Autodesk Fusion 360 part; units mm, degrees
sketch "Skizze1" plane through (0, 0, 0) normal (0, 0, 1) x (1, 0, 0)
  circle A0 centre (0, 0) radius 24.75
  circle A1 centre (0, 0) radius 21.75
  line L0 (-17.5, 13.5) -> (17.5, 13.5)
  line L1 (17.5, 13.5) -> (17.5, -13.5)
  line L2 (17.5, -13.5) -> (-17.5, -13.5)
  line L3 (-17.5, -13.5) -> (-17.5, 13.5)
  line L4 (-40, 0) -> (50, 0) construction
  line L5 (0, 45.7661) -> (0, -44.2339) construction
  line L6 (-16.0234, 16.5) -> (16.0234, 16.5)
  line L7 (20.5, 10.4283) -> (20.5, -10.4283)
  line L8 (16.0234, -16.5) -> (-16.0234, -16.5)
  line L9 (-20.5, -10.4283) -> (-20.5, 10.4283)
  arc A2 (6.5, 16.5) -> (-6.5, 16.5) centre (0, 16.5) ccw
  arc A3 (-6.6213, -16.5) -> (6.3787, -16.5) centre (-0.1213, -16.5) ccw
  arc A4 (-21.6357, 2.2272) -> (-21.6357, -2.2272) centre (-20.5, 0) ccw
  arc A5 (21.6357, -2.2272) -> (21.6357, 2.2272) centre (20.5, 0) ccw
  circle A6 centre (0, 0) radius 23
  line L10 (-14.5, -7.5) -> (14.5, -7.5)
  line L11 (14.5, -7.5) -> (14.5, 7.5)
  line L12 (14.5, 7.5) -> (-14.5, 7.5)
  line L13 (-14.5, 7.5) -> (-14.5, -7.5)
  line L14 (-15.5, 10.5) -> (15.5, 10.5)
  line L15 (15.5, 10.5) -> (15.5, -10.5)
  line L16 (15.5, -10.5) -> (-15.5, -10.5)
  line L17 (-15.5, -10.5) -> (-15.5, 10.5)
  dimension "d1" = 49.5
  dimension "d3" = 3
  dimension "d4" = 27
  dimension "d5" = 35
  dimension "d6" = 3
  dimension "d7" = 3
  dimension "d8" = 3
  dimension "d9" = 3
  dimension "d18" = 46
  dimension "d19" = 29
  dimension "d20" = 15
  dimension "d27" = 3
  dimension "d28" = 3
  dimension "d29" = 2
  dimension "d30" = 2
  dimension "d40" = 33
extrude "Extrusion5" add sketch "Skizze1" along normal blind 3 contours A1 L7 | A1 A5 | A1 L1 L7 | A1 L0 L1 L6 L7 A6 | A1 L1 L2 L7 L8 A6 | A1 L0 L6 | A1 L2 L8 | A1 L0 L3 L6 L9 A6 | A1 A2 | A1 A3 | A1 L2 L3 L8 L9 A6 | A1 L6 A2 | A1 L3 L9 | A1 L8 A3 | A1 L9 | A1 A4 picked at (0.4894, 18.2335) picked at (-0.6234, -18.2297)
extrude "Extrusion6" add sketch "Skizze1" along normal up to surface (1.5 mm away) from surface at 1.5 contours A1 L0 L1 L2 L3
hole "Bohrung1" at (0, 16.5, 0) at (20.5, 0, 0) at (-0.1213, -16.5, 0) at (-20.5, 0, 0) direction (0, 0, 1) diameter 2.5 end through all
fillet "Abrundung1" radius 7 4 edges at (-6.6213, -16.5, 1.5) (6.3787, -16.5, 1.5) (6.5, 16.5, 1.5) (-6.5, 16.5, 1.5)
Input: part model. Units: mm. Frame: model coordinates. A direction names the side the tool comes from. Give positions to 0.01 mm unless a question says otherwise; leave off trailing zeros. Order: outer loops, then holes, each group sorted by start corner. A loop starts at its lowest first (then second) coordinate and runs counter-clockwise, first axis right, second up.
Q1. Section B-B on x = 9. Output: boundary loops of the cut face in (y, z).
Checked values:
outline: (-16.93, 0) - (-13.5, 0) - (-13.5, 1.5) - (-10.5, 1.5) - (-10.5, 3) - (-16.93, 3) - close; (10.5, 1.5) - (13.5, 1.5) - (13.5, 0) - (16.98, 0) - (16.98, 3) - (10.5, 3) - close
Q2. Section C-C on y = -5.5. Output: boundary loops of the cut face in (x, z), and give its area (3 significant figures).
Checked values:
outline: (-21.04, 0) - (-17.5, 0) - (-17.5, 1.5) - (-15.5, 1.5) - (-15.5, 3) - (-21.04, 3) - close; (15.5, 1.5) - (17.5, 1.5) - (17.5, 0) - (21.04, 0) - (21.04, 3) - (15.5, 3) - close
area: 27.3 mm2
Q3. Section D-D on z = 0.7. State how many separate pieces and enclosed holes the cut face has, and give its area (3 significant figures).
Checked values:
separate pieces: 1
enclosed holes: 5
area: 520 mm2
Q4. Ray query, probe 1 along X at (y, z) = (0, 1.65); probe 2 along X at (y, z) = (7.5, 2.1); probe 3 along Y at (x, z) = (13, 1.4). Return the intervals inside material, ascending.
Checked values:
probe 1: x = -23 to -21.75, -19.25 to -15.5, 15.5 to 19.25, 21.75 to 23
probe 2: x = -20.5 to -15.5, 15.5 to 20.5
probe 3: y = -16.5 to -13.5, 13.5 to 16.5
Q5. Section A-A on y = 0. Output: boundary loops of the cut face in (x, z).
Checked values:
outline: (-23, 0) - (-21.75, 0) - (-21.75, 3) - (-23, 3) - close; (-19.25, 0) - (-17.5, 0) - (-17.5, 1.5) - (-15.5, 1.5) - (-15.5, 3) - (-19.25, 3) - close; (15.5, 1.5) - (17.5, 1.5) - (17.5, 0) - (19.25, 0) - (19.25, 3) - (15.5, 3) - close; (21.75, 0) - (23, 0) - (23, 3) - (21.75, 3) - close
Q6. Set-up query: faces 1 (the flat face through (-20.5, 9, 1)), 2 (the flat face through (-14, -16.5, 1)), 3 (the flat face through (20.5, 9, 1)). Return all of +Z, -Z, +X, -X, +Y, -Y with unobstructed straight access to the full face (end or side cutting, diameter ignored); none if empty.
Checked values:
face 1: +Z, -Z, -X, +Y
face 2: +Z, -Z, -X, -Y
face 3: +Z, -Z, +X, +Y
Q7. Draft query along Y for faces 4 (the cylindrical face through (-21.21, -4.82, 1.48)), 5 (the flat face through (-14, 16.5, 1)), 6 (the cylindrical face through (-0.18, -17.75, 1.52)). Return one class per face: +Y half, -Y half, draft (parallel to the pull), parting line (faces both ways), or undercut.
Checked values:
face 4: -Y half
face 5: +Y half
face 6: undercut
Q8. Contact query for flat-ended pins moving along their axis: pin 1 Ø1.5 at (y, z) = (8.5, 2) entering from -X; pin 2 Ø0.8 at (x, z) = (2, 2) entering from -Y; pin 3 Ø1.6 at (y, z) = (4.5, 2.5) entering from +X; pin 4 Ø2 at (x, y) = (-20.5, 0) entering from -Z. Output: stop coordinate, or through.
Checked values:
pin 1: stops at x = -20.5
pin 2: stops at y = -22.77
pin 3: stops at x = 21.43
pin 4: passes through
